Part model, mm, in its own coordinate system. A direction names the side the tool comes from. Give positions to 0.01 mm unless a question says otherwise; leave off trailing zeros. Loops run counter-clockwise (first coordinate to the right, second up) from the corner with the lowest first, then second, coordinate; pieces in that order, holes last. Notation, with made-up numbers: M 14,77 L 41,77 A32 cw 41,115 Z; hole C -38,3.5 d11. An arc over 180 degrees is marked long. Answer in a Markdown table with one row per item.
Autodesk Fusion 360 part; units mm, degrees
sketch "Schizzo1" plane through (0, 0, 0) normal (1, 0, 0) x (0, 1, 0)
  line L0 (0, 0) -> (0, 13.6)
  line L1 (0, 13.6) -> (4, 13.6)
  line L2 (4, 13.6) -> (4, 6.6)
  line L3 (4, 6.6) -> (6, 6.6)
  line L4 (6, 6.6) -> (6, 5.6)
  line L5 (6, 5.6) -> (4, 1)
  line L6 (4, 1) -> (4, 0)
  line L7 (4, 0) -> (0, 0)
  line L8 (0, 0) -> (0, -9.2) construction
  line L9 (0, -9.2) -> (10, -9.2) construction
  line L10 (0, -4) -> (10, -4) construction
  line L11 (0, 6.8) -> (10, 6.8) construction
  dimension "d1" = 8
  dimension "d2" = 8
  dimension "d3" = 7
  dimension "d4" = 10.8
  dimension "d5" = 16
  dimension "d6" = 0.2
  dimension "d7" = 10
  dimension "d8" = 2
  dimension "d10" = 4
  dimension "d11" = 1
  dimension "d12" = 1
revolve "Rivoluzione1" add sketch "Schizzo1" angle 360 about axis through (0, 0, 0) along (0, 0, 1)
chamfer "Smusso1" distance 0.6 angle 45 1 edges at (-3.7293, 1.4465, 13.6)
component "Component" placed x (1, 0, 0) y (0, 1, 0) z (0, 0, 1) at (0, 0, 0)
(1) Saw through at A-A (x = 0). Write the cut outline in (y, z).
Recorded:
| item | result |
|---|---|
| outline | M -6,5.6 L -4,1 L -4,0 L 4,0 L 4,1 L 6,5.6 L 6,6.6 L 4,6.6 L 4,13 L 3.4,13.6 L -3.4,13.6 L -4,13 L -4,6.6 L -6,6.6 Z |
(2) Drill centre lines: line 1 along Y through (x, z) = (-0.25, 5.5); line 2 along X through (y, z) = (2.5, 10.5); line 3 along X through (y, z) = (2.75, 12.25). Where is each one in solid material? Low to high.
Recorded:
| item | result |
|---|---|
| line 1 | y = -5.95 to 5.95 |
| line 2 | x = -3.12 to 3.12 |
| line 3 | x = -2.9 to 2.9 |
(3) Saw through at C-C (z = 6). Write the cut outline in (x, y), plus the area to 3 significant figures.
Recorded:
| item | result |
|---|---|
| outline | C 0,0 d12 |
| area | 113 mm^2 |
(4) Which spindle directions (+Z, -Z, +X, -X, +Y, -Y) get a long thin tool onto all of the face, cutting with end or side? Do faces 1 (the face through (0, 0, 13.6)), 2 (the face through (-3.905, -0.867, 0.493)), 3 (the face through (-3.905, -0.867, 9.755)). Say none if no direction does.
Recorded:
| item | result |
|---|---|
| face 1 | +Z, +X, -X, +Y, -Y |
| face 2 | -Z |
| face 3 | +Z |
(5) Pin check, flat tips, straight feed: pin 1 Ø5 at (x, y) = (4, -3) entering from +Z; pin 2 Ø1 at (y, z) = (4, 10.5) entering from +X; pin 3 Ø2 at (y, z) = (1.5, 4) entering from -X; pin 4 Ø1 at (y, z) = (0, 4.5) entering from +X. Stop position of each tip, or through.
Recorded:
| item | result |
|---|---|
| pin 1 | stops at z = 13.6 |
| pin 2 | stops at x = 1.94 |
| pin 3 | stops at x = -5.6 |
| pin 4 | stops at x = 5.74 |
(6) Saw through at D-D (z = 1.5). Write the cut outline in (x, y), plus the area to 3 significant figures.
Recorded:
| item | result |
|---|---|
| outline | C 0,0 d8.43 |
| area | 55.9 mm^2 |
